from build123d import *

# Parameters (mm, degrees)
SKETCH_W          = 60
SKETCH_H          = 10
PAD_DEPTH         = 40
PAD001_DEPTH      = 40
PAD002_DEPTH      = 9
PAD002_DEPTH_BACK = 9
SKETCH003_R       = 5
POCKET_DEPTH      = 18
POCKET001_DEPTH   = 40
POCKET002_DEPTH   = 10


with BuildPart() as part:
    # Sketch → Pad (new body)
    with BuildSketch(Plane.XZ):
        Rectangle(SKETCH_W, SKETCH_H)
    extrude(amount=PAD_DEPTH)

    # Sketch001 → Pad001 (join)
    with BuildSketch(Plane.XZ):
        with BuildLine():
            Line((-19.816975, 4.999952), (-19.816975, 20))
            ThreePointArc((20.183025, 19.999952), (0.183049, 40), (-19.816975, 20))
            Line((20.183025, 19.999952), (20.183025, 4.999952))
            Line((20.183025, 4.999952), (-19.816975, 4.999952))
        make_face()
    extrude(amount=PAD001_DEPTH)

    # Sketch002 → Pad002 (join, two sides)
    with BuildSketch(Plane.YZ) as pad002_sk:
        with BuildLine():
            Line((-30, 25), (-30, 45))
            ThreePointArc((-10, 45), (-20, 55), (-30, 45))
            Line((-10, 45), (-10, 25))
            Line((-10, 25), (-30, 25))
        make_face()
    extrude(amount=PAD002_DEPTH)
    extrude(pad002_sk.sketch, amount=-PAD002_DEPTH_BACK)

    # Sketch003 (on Face17 of Pad002) → Pocket (cut)
    with BuildSketch(Plane(origin=(9, 0, 0), x_dir=(0, 0, 1), z_dir=(1, 0, 0))):
        with Locations((45, 20)):
            Circle(SKETCH003_R)
    extrude(amount=-POCKET_DEPTH, mode=Mode.SUBTRACT)

    # Sketch004 (on Face12 of Pocket) → Pocket001 (cut)
    with BuildSketch(Plane.XZ.offset(40)):
        with BuildLine():
            ThreePointArc((-2, 32.845233), (0, 7), (2, 32.845233))
            Line((2, 57.141209), (2, 32.845233))
            Line((-2, 57.141209), (2, 57.141209))
            Line((-2, 32.845233), (-2, 57.141209))
        make_face()
    extrude(amount=-POCKET001_DEPTH, mode=Mode.SUBTRACT)

    # Sketch005 (on Face8 of Pocket001) → Pocket002 (cut)
    with BuildSketch(Plane(origin=(0, 0, 5), x_dir=(-1, 0, 0), z_dir=(0, 0, 1))):
        with BuildLine():
            ThreePointArc((-28, 8), (-25, 5), (-22, 8))
            Line((-22, 8), (-22, 32))
            ThreePointArc((-22, 32), (-25, 35), (-28, 32))
            Line((-28, 8), (-28, 32))
        make_face()
        with BuildLine():
            ThreePointArc((22, 8), (25, 5), (28, 8))
            Line((28, 8), (28, 32))
            ThreePointArc((28, 32), (25, 35), (22, 32))
            Line((22, 8), (22, 32))
        make_face()
    extrude(amount=-POCKET002_DEPTH, mode=Mode.SUBTRACT)


solid = part.part
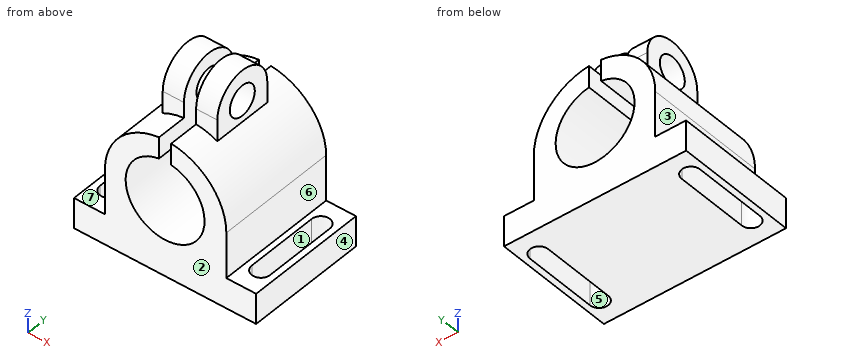
Input: part model. Units: mm. Frame: model coordinates. Face numbers are marked on the shaded views. A direction names the side the tool comes from. Coordinates: 2 decimals unless noted, no trailing zeros. Loops run counter-clockwise (first coordinate to the right, second up) from the corner with the lowest first, then second, coordinate; pieces in that order, holes last. Notation, with made-up numbers: (32, 30.5) -> (39, 30.5) arc R19 cw to (39, 48.5) -> close; hole circle Ø10 at (-2, -4). An arc over 180 degrees is marked (long way). Write item = value, one per line. Start each with the question number.
Item 1: Cut plane A-A, the plane z = 51. Return loops of the section in (x, y).
Item 2: First-contact query: P1, Ø3, axis at x = -27, y = -20, coming from the +Z side; P2, Ø2, axis at x = -5, z = 42, coming from the -Y side; P3, Ø17.5, axis at y = -13.5, z = 47.5, coming from the -X side; P4, Ø15.5, axis at x = 0, z = 20, coming from the +Y side. Flat tips, straight axial feed; report the tip coordinate or a pass-through.
Item 3: Mould query, pull axis X, two halves, no side actions, for the marked faces 1, 2, 3 and 4. Classes: pulls with the +X half, pulls with the -X half, needs draft (parallel to the pull), parting line crosses it, or undercut.
Item 4: Cut plane B-B, the plane x = -3. Return loops of the section in (y, z), plus the area to 3 significant figures.
Item 5: Reachability of the marked faces 5, 6 and 7 from +Z, -Z, +X, -X, +Y, -Y: full face, straight path, thin tool, end or side. Return the list, or none.
Item 6: Cut plane D-D, the plane x = -25. Return loops of the section in (y, z), plus the area to 3 significant figures.
Item 7: Material intervals for line 1 (X direction, y = -17, z = -2); line 2 (Z direction, x = -5.5, y = -20); line 3 (Z direction, x = 4.5, y = -20), sorted ascending.
Item 8: Cut plane C-C, the plane y = -21. Count the separate pieces of the cut face and the enclosed holes in it, plus the area to 3 significant figures.
Ans:
q1.outline = (-9, -28) -> (-2, -28) -> (-2, -12) -> (-9, -12) -> close; (2, -28) -> (9, -28) -> (9, -12) -> (2, -12) -> close
q2.P1 = 5
q2.P2 = -30
q2.P3 = -9
q2.P4 = through
q3.face_1 = undercut
q3.face_2 = needs draft
q3.face_3 = pulls with the -X half
q3.face_4 = pulls with the +X half
q4.outline = (-40, -5) -> (0, -5) -> (0, 7.35) -> (-40, 7.35) -> close; (-40, 32.65) -> (0, 32.65) -> (0, 39.75) -> (-10, 39.75) -> (-10, 45) arc R10 ccw to (-30, 45) -> (-30, 39.75) -> (-40, 39.75) -> close; hole circle Ø10 at (-20, 45)
q4.area = 962 mm²
q5.face_5 = +Z, -Z
q5.face_6 = +Z, +X, +Y, -Y
q5.face_7 = +Z, -X, +Y, -Y
q6.outline = (-40, -5) -> (-35, -5) -> (-35, 5) -> (-40, 5) -> close; (-5, -5) -> (0, -5) -> (0, 5) -> (-5, 5) -> close
q6.area = 100 mm²
q7.line_1 = -30 to -28, -22 to 22, 28 to 30
q7.line_2 = -5 to 8.22, 31.78 to 40, 50 to 55
q7.line_3 = -5 to 7.8, 32.2 to 40, 50 to 55
q8.separate_pieces = 5
q8.enclosed_holes = 0
q8.area = 1,230 mm²
